```python
from build123d import *

# Parameters (mm, degrees)
BOSS_EXTRUDE1_DEPTH = 8.525
SKETCH2_W           = 0.5
SKETCH2_H           = 7
BOSS_EXTRUDE2_DEPTH = 0.25
SKETCH3_W           = 2.6
SKETCH3_H           = 6
BOSS_EXTRUDE3_DEPTH = 0.01


with BuildPart() as part:
    # Sketch1 → Boss-Extrude1 (new, symmetric)
    with BuildSketch(Plane(origin=(0, 0, 0), x_dir=(0, 0, -1), z_dir=(1, 0, 0))):
        Polygon((-3, 0.515), (3, 0.515), (4.6, 1.125), (5.6, 1.125), (5.6, -1.125), (-5.6, -1.125), (-5.6, 1.125), (-4.6, 1.125), align=None)
    extrude(amount=BOSS_EXTRUDE1_DEPTH, both=True)

    # Sketch2 → Boss-Extrude2 (add)
    with BuildSketch(Plane(origin=(0, 0.515, 0), x_dir=(1, 0, 0), z_dir=(0, 1, 0))):
        with Locations((-7.86, 0)):
            Rectangle(SKETCH2_W, SKETCH2_H)
        with Locations((-3.93, 0)):
            Rectangle(SKETCH2_W, SKETCH2_H)
        Rectangle(SKETCH2_W, SKETCH2_H)
        with Locations((3.93, 0)):
            Rectangle(SKETCH2_W, SKETCH2_H)
        with Locations((7.86, 0)):
            Rectangle(SKETCH2_W, SKETCH2_H)
    extrude(amount=BOSS_EXTRUDE2_DEPTH)

    # Sketch3 → Boss-Extrude3 (add)
    with BuildSketch(Plane(origin=(0, 0.515, 0), x_dir=(1, 0, 0), z_dir=(0, 1, 0))):
        with Locations((-5.895, 0)):
            Rectangle(SKETCH3_W, SKETCH3_H)
        with Locations((-1.965, 0)):
            Rectangle(SKETCH3_W, SKETCH3_H)
        with Locations((1.965, 0)):
            Rectangle(SKETCH3_W, SKETCH3_H)
        with Locations((5.895, 0)):
            Rectangle(SKETCH3_W, SKETCH3_H)
    extrude(amount=BOSS_EXTRUDE3_DEPTH)


solid = part.part
```
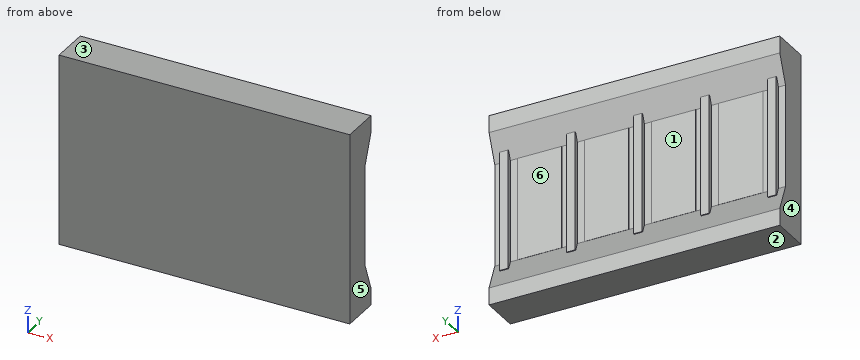
Can you work these out from the model? Positions are in its coordinate system, mm. Face numbers are marked on the shaded views. A direction names the side the tool comes from. Give positions to 0.01 mm unless a question says otherwise; leave off trailing zeros. Write each loop counter-clockwise with the first axis right and the second up, starting at its lowest first coordinate (ties: lowest second). Pieces come first, ordered by that corner, then holes. Notation, with made-up numbers: (49, 27.25) -> (68, 27.25) arc R22 cw to (68, 56.25) -> close; hole circle Ø9 at (5, 60.5). An arc over 180 degrees is marked (long way). Write item = value, one per line.
(1) Thinking about a two-plate mould opening in X: for the marked faces 3, 4, 5 and 6, which applies, released by +X, released by -X, zero draft, split by the parting line, or undercut?
Worked out:
face_3 = zero draft
face_4 = released by -X
face_5 = released by +X
face_6 = undercut
(2) I'm going to push flat-ended pins straight in: P1, Ø1, axis at x = -6, z = -4, coming from the +Y side; P2, Ø1, axis at x = -5, z = -1, coming from the +Y side (3 decimals); P3, Ø3, axis at x = -1.5, z = 2.5, coming from the +Y side. Where does each tip first touch, or does it pass through?
Worked out:
P1 = 1.09
P2 = 0.525
P3 = 0.9
(3) Suppose I cut it at C-C on z = 4. Write out the boundary of the cut face in (x, y) (3 decimals), then the cut area to 3 significant figures.
Worked out:
outline = (-8.525, -1.125) -> (8.525, -1.125) -> (8.525, 0.896) -> (-8.525, 0.896) -> close
area = 34.5 mm^2
(4) I need wall thicknesses on probe 1 along Y at (x, z) = (-2, -2.25) (3 decimals); probe 2 along Y at (x, z) = (4, 0) (3 decimals). Which ranges of each line are inside material? Lowest first, please. Write a range as from..to.
Worked out:
probe_1 = -1.125..0.525
probe_2 = -1.125..0.765
(5) Suppose I cut it at D-D on x = -6. Write out the boundary of the cut face in (y, z) (3 decimals).
Worked out:
outline = (-1.125, -5.6) -> (1.125, -5.6) -> (1.125, -4.6) -> (0.515, -3) -> (0.525, -3) -> (0.525, 3) -> (0.515, 3) -> (1.125, 4.6) -> (1.125, 5.6) -> (-1.125, 5.6) -> close
(6) For the marked faces 1 and 2, which set-ups out of +Z, -Z, +X, -X, +Y, -Y let a thin tool reach every point of the face, with its end or its side?
Worked out:
face_1 = +Y
face_2 = -Z, +X, -X, +Y, -Y
(7) Suppose I cut it at B-B on x = -3.5. Write out the boundary of the cut face in (y, z) (3 decimals).
Worked out:
outline = (-1.125, -5.6) -> (1.125, -5.6) -> (1.125, -4.6) -> (0.515, -3) -> (0.515, 3) -> (1.125, 4.6) -> (1.125, 5.6) -> (-1.125, 5.6) -> close
(8) Suppose I cut it at A-A on x = 0. Write out the boundary of the cut face in (y, z) (3 decimals), then the cut area to 3 significant figures.
Worked out:
outline = (-1.125, -5.6) -> (1.125, -5.6) -> (1.125, -4.6) -> (0.706, -3.5) -> (0.765, -3.5) -> (0.765, 3.5) -> (0.706, 3.5) -> (1.125, 4.6) -> (1.125, 5.6) -> (-1.125, 5.6) -> close
area = 22.2 mm^2
